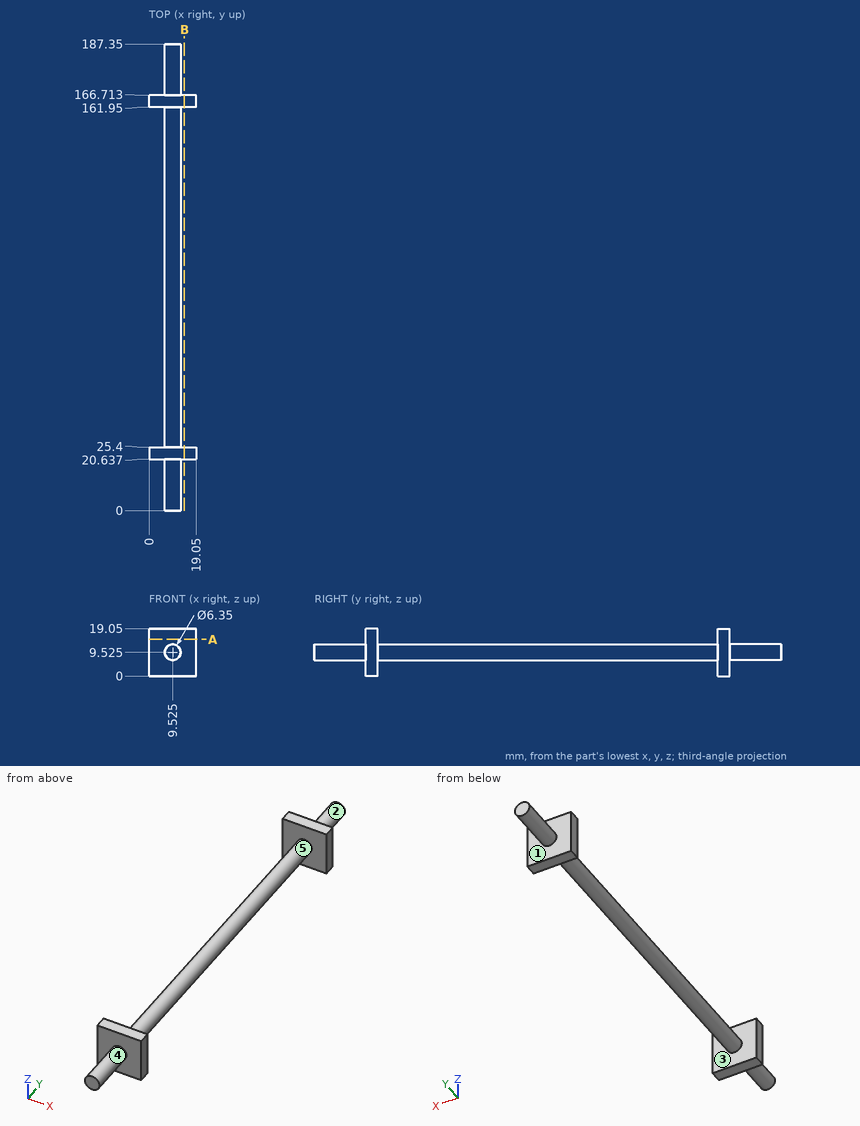
Study the drawing (mm; zero at the part's minimum x, y, z) and answer. A direction names the side the tool comes from. Give positions to 0.01 mm unless a question says otherwise; leave off trailing zeros. Loops run counter-clockwise (first coordinate to the right, second up) from the corner with the lowest first, then second, coordinate; pieces in that order, holes last. Notation, with made-up numbers: (0, 5) - (57, 5) arc R20 cw to (57, 19) - close; hole circle Ø5 at (-3.5, 3.5). An arc over 180 degrees is marked (long way). Use CSV: the item, a comma, the result in double quotes. Start each with the question number.
(1) Each of these flat-tipped pins is pushed along its axis until it touches: pin 1 (10 mm diameter, centred on x = 14, y = 96.5, fed in from -Z); pin 2 (4 mm diameter, centred on x = 4.5, z = 8, fed in from -Y); pin 3 (4 mm diameter, centred on x = 16, z = 11.5, fed in from +Y). Where does it stop, or does it pass through?
(2) Find the intervals of material crossed by L1, parallel to Y at x = 7.75, z = 15.5; L2, parallel to X at y = 150.5, z = 6.75 (1 decimal); L3, parallel to X at y = 106.5, z = 7.5, in increasing order.
(3) Find section B-B, the plane x = 14.25. Determine the outline of the cut face in (y, z).
(4) Find section A-A, the plane z = 14.75. Determine the outline of the cut face in (x, y).
(5) A tool of negligible diameter and unlimited length cuts with its end or side. For the marked faces 4 and 5, from which of +Z, -Z, +X, -X, +Y, -Y can it reach the whole face along a straight path? Write none if from no direction.
(6) Determine the mould class of the marked faces 1, 2 and 3 for opening direction Y: released by +Y, released by -Y, zero draft, split by the parting line, or undercut.
Results found:
1,pin 1,"z = 6.35"
1,pin 2,"y = 20.64"
1,pin 3,"y = 166.71"
2,L1,"20.64 to 25.4, 161.95 to 166.71"
2,L2,"8 to 11.1"
2,L3,"7.08 to 11.97"
3,outline,"(20.64, 0) - (25.4, 0) - (25.4, 19.05) - (20.64, 19.05) - close; (161.95, 0) - (166.71, 0) - (166.71, 19.05) - (161.95, 19.05) - close"
4,outline,"(0, 20.64) - (19.05, 20.64) - (19.05, 25.4) - (0, 25.4) - close; (0, 161.95) - (19.05, 161.95) - (19.05, 166.71) - (0, 166.71) - close"
5,face 4,"-Y"
5,face 5,"none"
6,face 1,"released by +Y"
6,face 2,"zero draft"
6,face 3,"undercut"
